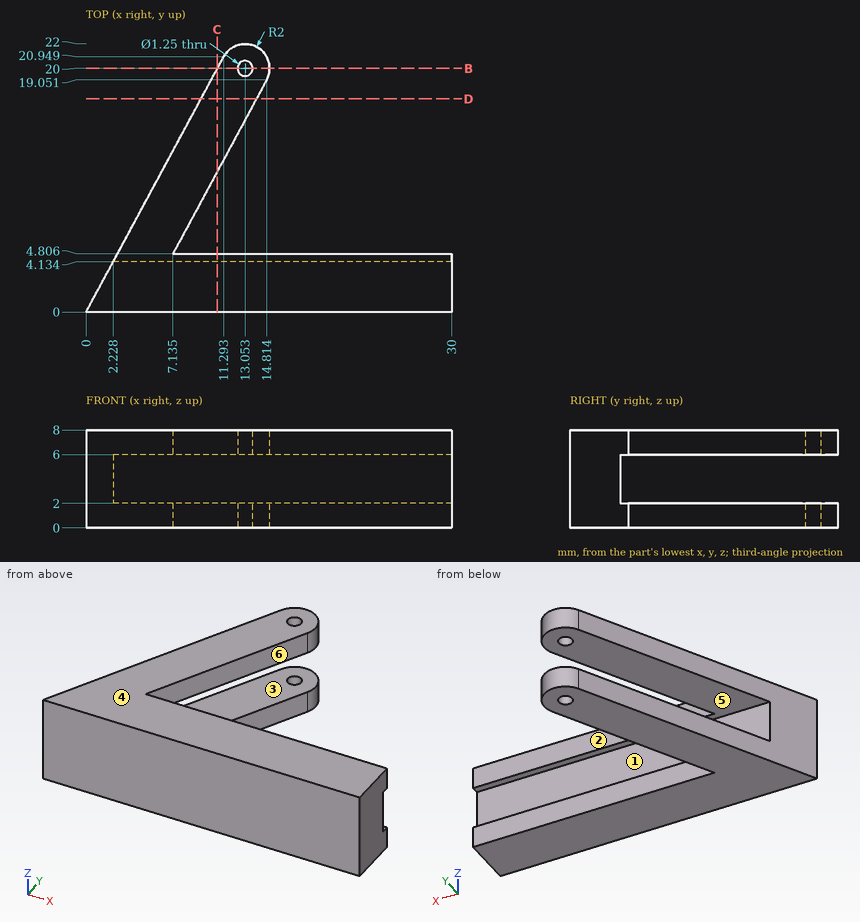
Geometry: see drawing. Coordinates: mm, zero at the bounding-box minimum. A direction names the side the tool comes from. Give positions to 0.01 mm unless a question says otherwise; leave off trailing zeros. Order: outer loops, then holes, each group sorted by start corner. A loop starts at its lowest first (then second) coordinate and runs counter-clockwise, first axis right, second up. Notation, with made-up numbers: (-28, -35.5) - (29, -35.5) arc R18 ccw to (29, -6.5) - close; hole circle Ø8 at (79, 10). An arc over 180 degrees is marked (long way). Write each question's results on one line, items separated by ' | '.
Item 1: Section C-C (x = 10.75). Return loops of the section in (y, z).
A:
outline: (0, 0) - (4.81, 0) - (4.81, 2) - (4.13, 2) - (4.13, 6) - (4.81, 6) - (4.81, 8) - (0, 8) - close; (11.51, 0) - (19.94, 0) - (19.94, 2) - (11.51, 2) - close; (11.51, 6) - (19.94, 6) - (19.94, 8) - (11.51, 8) - close
Item 2: Contact query for a flat-ended pin moving along its axis: pin 1 Ø4 at (x, z) = (17.5, 1) entering from +Y. Output: stop coordinate, or through.
A:
pin 1: stops at y = 4.81
Item 3: Section B-B (y = 20). Return loops of the section in (x, z), and give its area (3 significant figures).
A:
outline: (10.78, 0) - (12.43, 0) - (12.43, 2) - (10.78, 2) - close; (10.78, 6) - (12.43, 6) - (12.43, 8) - (10.78, 8) - close; (13.68, 0) - (15.05, 0) - (15.05, 2) - (13.68, 2) - close; (13.68, 6) - (15.05, 6) - (15.05, 8) - (13.68, 8) - close | area: 12.1 mm^2
Item 4: Material intervals for line 1 along Z through (x, y) = (7.75, 13.5); line 2 along Y through (x, z) = (12.5, 7.75) (1 decimal); line 3 along Y through (x, z) = (21.75, 7.5), sorted ascending.
A:
line 1: z = 0 to 2, 6 to 8 | line 2: y = 0 to 4.8, 14.8 to 19.7, 20.3 to 21.9 | line 3: y = 0 to 4.81
Item 5: Access query for the marked faces 4, 5 and 6. Directions: +Z, -Z, +X, -X, +Y, -Y. A direction counts if a zero-diameter tool reaches every point of the face in a straight line with its end or side. Return the directions, or none.
A:
face 4: +Z, +X, -X, +Y, -Y | face 5: +X, -X, +Y | face 6: +Z, -Z, +X
Item 6: Section D-D (y = 17.5). Return loops of the section in (x, z).
A:
outline: (9.43, 0) - (13.98, 0) - (13.98, 2) - (9.43, 2) - close; (9.43, 6) - (13.98, 6) - (13.98, 8) - (9.43, 8) - close
Item 7: Draft query along Y for the marked faces 1, 2 and 3. Return one class per face: released by +Y, released by -Y, zero draft, split by the parting line, or undercut.
A:
face 1: released by +Y | face 2: undercut | face 3: zero draft
